Read the model definition and answer for the solid it produces. Units are mm, in the model's axes. Face numbers are marked on the shaded views. Give positions to 0.01 mm unless a question says otherwise; leave off trailing zeros. Order: outer loops, then holes, each group sorted by start corner. A loop starts at its lowest first (then second) coordinate and runs counter-clockwise, first axis right, second up. Notation, with made-up numbers: M -13.75,16.25 L -4.75,16.25 A17 cw -4.75,23.25 Z; hole C 73.5,-20 d3. An arc over 180 degrees is marked long. Write item = value, one per line. Start each with the question number.
from build123d import *

# Parameters (mm, degrees)
SKETCH2_W           = 63.5
SKETCH2_H           = 12.7
BOSS_EXTRUDE1_DEPTH = 44.45
BOSS_EXTRUDE2_DEPTH = 3.175
SKETCH2_2_W         = 63.5
SKETCH2_2_H         = 12.7
BOSS_EXTRUDE3_DEPTH = 3.175
BOSS_EXTRUDE4_DEPTH = 3.175


with BuildPart() as part:
    # Sketch2 → Boss-Extrude1 (new body)
    with BuildSketch(Plane.XY):
        with Locations((-21.607638889, 1.984375)):
            Rectangle(SKETCH2_W, SKETCH2_H)
    extrude(amount=BOSS_EXTRUDE1_DEPTH)

    # Sketch3 → Boss-Extrude2 (add)
    with BuildSketch(Plane(origin=(0, 8.334375, 0), x_dir=(1, 0, 0), z_dir=(0, 1, 0))):
        with BuildLine():
            Line((27.384230149, -21.096568897), (24.686230398, -41.471557028))
            ThreePointArc((24.686230398, -41.471557028), (19.660883481, -45.321643523), (15.810796986, -40.296296607))
            Line((15.810796986, -40.296296607), (18.234581428, -20.32))
            ThreePointArc((18.234581428, -20.32), (18.251088657, -19.930319533), (18.300492073, -19.543431103))
            ThreePointArc((18.300492073, -19.543431103), (-0.851865875, 7.879150717), (-28.517114145, -10.920978184))
            ThreePointArc((-28.517114145, -10.920978184), (-33.930101581, -14.549040236), (-37.558163632, -9.136052801))
            ThreePointArc((-37.558163632, -9.136052801), (0.817302189, 16.942285518), (27.384230149, -21.096568897))
        make_face()
    extrude(amount=BOSS_EXTRUDE2_DEPTH)

    # Sketch2<2> → Boss-Extrude3 (add)
    with BuildSketch(Plane.XY):
        with Locations((-21.607638889, 1.984375)):
            Rectangle(SKETCH2_2_W, SKETCH2_2_H)
    extrude(amount=BOSS_EXTRUDE3_DEPTH)

    # Sketch6 → Boss-Extrude4 (add)
    with BuildSketch(Plane(origin=(0, 8.334375, 0), x_dir=(1, 0, 0), z_dir=(0, 1, 0))):
        with BuildLine():
            Line((-71.134197224, -21.655068851), (-67.914165266, -41.469070044))
            ThreePointArc((-67.914165266, -41.469070044), (-63.143827484, -44.92106421), (-59.671631072, -40.165410907))
            Line((-59.671631072, -40.165410907), (-62.760560613, -20.083656097))
            ThreePointArc((-62.760560613, -20.083656097), (-42.464339717, 7.82922996), (-14.386949358, -12.238802862))
            ThreePointArc((-14.386949358, -12.238802862), (-9.684746174, -15.772440511), (-5.918655002, -11.254269741))
            ThreePointArc((-5.918655002, -11.254269741), (-43.742205026, 16.249534133), (-71.134197224, -21.655068851))
        make_face()
    extrude(amount=BOSS_EXTRUDE4_DEPTH)


solid = part.part
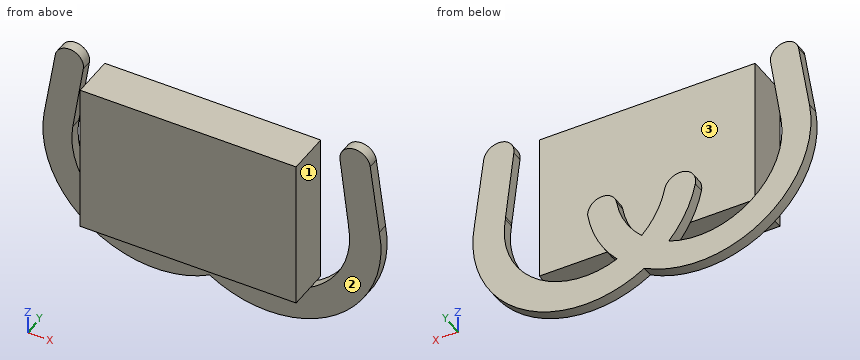
1) Find section A-A on x = 7. Determine the outline of the cut face in (y, z), plus the area to 3 significant figures.
2) Each of these flat-tipped pins is pushed along its axis until it touches: P1, Ø4, axis at y = 3, z = 16, coming from the -X side; P2, Ø4, axis at x = -9, y = 5, coming from the -Z side; P3, Ø10, axis at x = -60, z = 29, coming from the -Y side. Where does it stop, or does it pass through?
3) Find section C-C on y = 9.75. Determine the outline of the cut face in (x, z), plus the area to 3 significant figures.
4) Find section D-D on x = -16.5. Determine the outline of the cut face in (y, z), plus the area to 3 significant figures.
5) For a pull along X with two mould halves and no side action, classify the marked faces 1, 2 and 3 as pulls with the +X half, pulls with the -X half, needs draft (parallel to the pull), parting line crosses it, or undercut.
6) Find section B-B on z = 18. Determine the outline of the cut face in (x, y).
7) Find the intervals of material crossed by probe 1 along X at (y, z) = (-2.25, 35); probe 2 along Z at (x, y) = (-3, 3.75); probe 3 along Y at (x, z) = (-41, 0.5), in increasing order. Write a range as [from, to].
Numbers:
q1.outline = M -4.37,0 L 8.33,0 L 8.33,44.45 L -4.37,44.45 Z; M 8.33,-15.17 L 11.51,-15.17 L 11.51,-4.93 L 8.33,-4.93 Z
q1.area = 597 mm2
q2.P1 = -53.36
q2.P2 = 0
q2.P3 = 8.33
q3.outline = M -71.13,21.66 A33.02 ccw -22.56,-12.54 A33.02 ccw 27.38,21.1 L 24.69,41.47 A4.48 ccw 15.81,40.3 L 18.23,20.32 A4.61 ccw 18.3,19.54 A23.8 cw -14.56,-6.34 A33.02 ccw -5.92,11.25 A4.27 ccw -14.39,12.24 A24.5 cw -21.78,-1.51 A23.8 cw -28.52,10.92 A4.61 ccw -37.56,9.14 A33.02 ccw -29.75,-6.51 A24.5 cw -62.76,20.08 L -59.67,40.17 A4.17 ccw -67.91,41.47 Z
q3.area = 1,980 mm2
q4.outline = M -4.37,0 L 8.33,0 L 8.33,-15.48 L 11.51,-15.48 L 11.51,5.65 L 8.33,5.65 L 8.33,44.45 L -4.37,44.45 Z
q4.area = 632 mm2
q5.face_1 = pulls with the +X half
q5.face_2 = needs draft
q5.face_3 = undercut
q6.outline = M -71.52,8.33 L -62.99,8.33 L -62.99,11.51 L -71.52,11.51 Z; M -53.36,-4.37 L 10.14,-4.37 L 10.14,8.33 L -53.36,8.33 Z; M 18.51,8.33 L 27.76,8.33 L 27.76,11.51 L 18.51,11.51 Z
q7.probe_1 = [-53.36, 10.14]
q7.probe_2 = [0, 44.45]
q7.probe_3 = [-4.37, 8.33]
